Here's the drawing with two shaded views (mm, measured from the low corner). I have some questions. A direction names the side the tool comes from. Coordinates: 2 decimals unless noted, no trailing zeros. Order: outer loops, then holes, each group sorted by start corner. A loop starts at its lowest first (then second) coordinate and runs counter-clockwise, first axis right, second up. Notation, with made-up numbers: (62.25, 19.5) -> (86.25, 19.5) arc R29 ccw to (86.25, 51.5) -> close; hole circle Ø8 at (40.25, 30). An arc over 180 degrees is marked (long way). One line per item, written item: value. Start each with the question number.
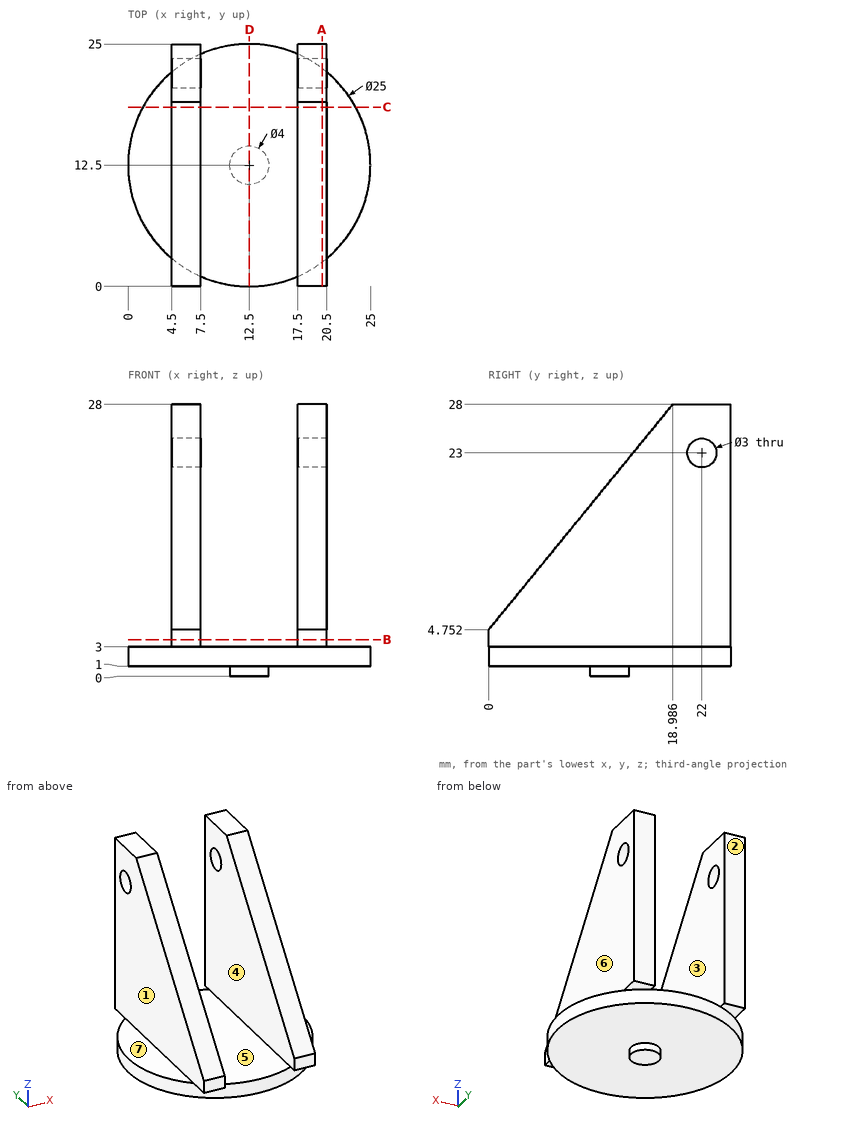
Q1. For the marked faces 1, 2 and 3, which set-ups out of +Z, -Z, +X, -X, +Y, -Y let a thin tool reach every point of the face, with its end or its side?
Q2. Imagine slicing it at D-D (x = 12.5). Write out the boundary of the cut face in (y, z).
Q3. Imagine slicing it at A-A (x = 20). Write out the boundary of the cut face in (y, z) (1 decimal), plus the area to 3 significant figures.
Q4. If we mould it in two halves opening along X, with no side actions, what happens to the marked faces 4, 5, 6 and 7? For each: +X half, -X half, draft (parallel to the pull), parting line (faces both ways), or undercut.
Q5. Imagine slicing it at C-C (y = 18.5). Write out the boundary of the cut face in (x, z) (1 decimal).
Q6. For P1, Ø8, axis at x = 12.5, y = 7, coming from the +Z side; P2, Ø2, axis at y = 12.5, z = 20.5, coming from the +X side; P3, Ø1.5, axis at y = 8, z = 7.5, coming from the -X side, each with a flat end and sliding along its axis, tell me the tip position at first contact or that it passes through.
Q7. Imagine slicing it at B-B (z = 3.75). Write out the boundary of the cut face in (x, y).
Q8. I need wall thicknesses on line 1 (X direction, y = 18.5, z = 13.75); line 2 (Z direction, x = 5.6, y = 22); line 3 (Z direction, x = 22.5, y = 7.25). Which ranges of each line are inside material? Lowest first, please.
Completed:
1. face 1: +Z, -X, +Y, -Y
1. face 2: +Z, -Z, +X, -X, +Y
1. face 3: +Z, +Y, -Y
2. outline: (0, 1) -> (10.5, 1) -> (10.5, 0) -> (14.5, 0) -> (14.5, 1) -> (25, 1) -> (25, 3) -> (0, 3) -> close
3. outline: (0, 3) -> (2.5, 3) -> (2.5, 1) -> (22.5, 1) -> (22.5, 3) -> (25, 3) -> (25, 28) -> (19, 28) -> (0, 4.8) -> close; hole circle Ø3 at (22, 23)
3. area: 437 mm2
4. face 4: undercut
4. face 5: undercut
4. face 6: +X half
4. face 7: draft
5. outline: (1.5, 1) -> (23.5, 1) -> (23.5, 3) -> (20.5, 3) -> (20.5, 27.4) -> (17.5, 27.4) -> (17.5, 3) -> (7.5, 3) -> (7.5, 27.4) -> (4.5, 27.4) -> (4.5, 3) -> (1.5, 3) -> close
6. P1: stops at z = 3
6. P2: stops at x = 20.5
6. P3: stops at x = 4.5
7. outline: (4.5, 0) -> (7.5, 0) -> (7.5, 25) -> (4.5, 25) -> close; (17.5, 0) -> (20.5, 0) -> (20.5, 25) -> (17.5, 25) -> close
8. line 1: x = 4.5 to 7.5, 17.5 to 20.5
8. line 2: z = 1 to 21.5, 24.5 to 28
8. line 3: z = 1 to 3
